For this review, take the finished solid that the model builds, in its own axes (mm). A direction names the side the tool comes from. Coordinates: 2 decimals unless noted, no trailing zeros. Loops run counter-clockwise (first coordinate to the right, second up) from the corner with the lowest first, then second, coordinate; pieces in that order, holes last. Notation, with made-up numbers: (-11.75, 43.25) -> (7.25, 43.25) arc R21 cw to (7.25, 62.25) -> close; hole circle Ø4 at (51.25, 57). An arc over 180 degrees is marked (long way). Use a Markdown table: item, result.
from build123d import *

# Parameters (mm, degrees)
SKETCH2_R           = 150.026309836
BOSS_EXTRUDE1_DEPTH = 7
SKETCH3_W           = 125
SKETCH3_H           = 115
BOSS_EXTRUDE2_DEPTH = 185
SKETCH4_W           = 315
SKETCH4_H           = 250
BOSS_EXTRUDE3_DEPTH = 11
SKETCH5_R           = 28.662420382
BOSS_EXTRUDE4_DEPTH = 790
SKETCH6_W           = 690
SKETCH6_H           = 450
BOSS_EXTRUDE5_DEPTH = 18
SKETCH7_R           = 29.971446918
BOSS_EXTRUDE6_DEPTH = 50
BOSS_EXTRUDE7_DEPTH = 22
BOSS_EXTRUDE8_DEPTH = 37
FILLET1_R           = 10


with BuildPart() as part:
    # Sketch2 → Boss-Extrude1 (new body)
    with BuildSketch(Plane(origin=(0, 0, 0), x_dir=(1, 0, 0), z_dir=(0, 1, 0))):
        with Locations(Location((0, 0, 0), (0, 0, 270))):
            Circle(SKETCH2_R)
    extrude(amount=-BOSS_EXTRUDE1_DEPTH)

    # Sketch3 → Boss-Extrude2 (add)
    with BuildSketch(Plane.XZ.offset(7)):
        Rectangle(SKETCH3_W, SKETCH3_H)
    extrude(amount=BOSS_EXTRUDE2_DEPTH)

    # Sketch4 → Boss-Extrude3 (add)
    with BuildSketch(Plane.XZ.offset(192)):
        Rectangle(SKETCH4_W, SKETCH4_H)
    extrude(amount=BOSS_EXTRUDE3_DEPTH)

    # Sketch5 → Boss-Extrude4 (add)
    with BuildSketch(Plane.XZ.offset(203)):
        with Locations(Location((0, 0, 0), (0, 0, 90))):
            Circle(SKETCH5_R)
    extrude(amount=BOSS_EXTRUDE4_DEPTH)

    # Sketch6 → Boss-Extrude5 (add)
    with BuildSketch(Plane.XZ.offset(993)):
        Rectangle(SKETCH6_W, SKETCH6_H)
    extrude(amount=BOSS_EXTRUDE5_DEPTH)

    # Sketch7 → Boss-Extrude6 (add)
    with BuildSketch(Plane.XZ.offset(1011)):
        with Locations(Location((-295, 175, 0), (0, 0, 270))):
            Circle(SKETCH7_R)
        with Locations(Location((-295, -175, 0), (0, 0, 270))):
            Circle(SKETCH7_R)
        with Locations(Location((295, 175, 0), (0, 0, 270))):
            Circle(SKETCH7_R)
        with Locations(Location((295, -175, 0), (0, 0, 270))):
            Circle(SKETCH7_R)
    extrude(amount=BOSS_EXTRUDE6_DEPTH)

    # Sketch11 → Boss-Extrude7 (add)
    with BuildSketch(Plane(origin=(0, -423, 0), x_dir=(-1, 0, 0), z_dir=(0, -1, 0))):
        Polygon((28.709807748, 0), (28.709807748, -80), (-171.290192252, -80), (-171.290192252, 80), (28.709807748, 80), align=None)
    extrude(amount=BOSS_EXTRUDE7_DEPTH)

    # Sketch12 → Boss-Extrude8 (add)
    with BuildSketch(Plane.XY.offset(80)):
        with BuildLine():
            Line((-77.568003655, -253), (28.662420382, -423))
            ThreePointArc((28.662420382, -423), (-109.452791637, -391.115212019), (-77.568003655, -253))
        make_face()
    boss_extrude8 = extrude(amount=-BOSS_EXTRUDE8_DEPTH)

    # Mirror1: Boss-Extrude8 across plane
    add(boss_extrude8.mirror(Plane.XY))

    # Fillet1
    fillet1_edges = [part.edges().sort_by_distance(p)[0] for p in [
        (-157.5, -197.5, 125),
        (-157.5, -197.5, -125),
        (157.5, -197.5, -125),
        (157.5, -197.5, 125),
    ]]
    fillet(fillet1_edges, radius=FILLET1_R)


solid = part.part
(1) Take a section at A-A on z = -175. Write out the cut boundary in (x, y), plus the area to 3 significant figures.
Found:
| item | result |
|---|---|
| outline | (-345, -1011) -> (-324.97, -1011) -> (-324.97, -1061) -> (-265.03, -1061) -> (-265.03, -1011) -> (265.03, -1011) -> (265.03, -1061) -> (324.97, -1061) -> (324.97, -1011) -> (345, -1011) -> (345, -993) -> (-345, -993) -> close |
| area | 18,400 mm^2 |
(2) Take a section at B-B on x = 295. Write out the cut boundary in (y, z).
Found:
| item | result |
|---|---|
| outline | (-1061, -204.97) -> (-1011, -204.97) -> (-1011, -225) -> (-993, -225) -> (-993, 225) -> (-1011, 225) -> (-1011, 204.97) -> (-1061, 204.97) -> (-1061, 145.03) -> (-1011, 145.03) -> (-1011, -145.03) -> (-1061, -145.03) -> close |
(3) Mouldability with a two-part tool opening along Z and no side actions: class faces 4 (the face through (-25.196, -336.81, 61.759)), 5 (the face through (92, -423, -1)), 6 (the face through (-1, -98, -57.5)) as pulls with the +Z half, pulls with the -Z half, needs draft (parallel to the pull), parting line crosses it, or undercut.
Found:
| item | result |
|---|---|
| face 4 | needs draft |
| face 5 | undercut |
| face 6 | pulls with the -Z half |
(4) For pin 1 Ø9 at (x, y) = (-59, -198.5) entering from -Z; pin 2 Ø8 at (x, z) = (149.5, 169.5) entering from -Y; pin 3 Ø17.5 at (y, z) = (-438, 15.5) entering from -X, all flat-tipped, find the tip position at first contact; note any pin that passes through.
Found:
| item | result |
|---|---|
| pin 1 | stops at z = -125 |
| pin 2 | stops at y = -1011 |
| pin 3 | stops at x = -28.71 |
(5) Take a section at D-D on x = -109.5. Write out the cut boundary in (y, z), plus the area to 3 significant figures.
Found:
| item | result |
|---|---|
| outline | (-1011, -225) -> (-993, -225) -> (-993, 225) -> (-1011, 225) -> close; (-391.04, -80) -> (-284.96, -80) -> (-284.96, -43) -> (-391.04, -43) -> close; (-391.04, 43) -> (-284.96, 43) -> (-284.96, 80) -> (-391.04, 80) -> close; (-203, -125) -> (-192, -125) -> (-192, 125) -> (-203, 125) -> close; (-7, -102.56) -> (0, -102.56) -> (0, 102.56) -> (-7, 102.56) -> close |
| area | 20,100 mm^2 |
(6) For line 1 along Y through (x, z) = (148, 53); line 2 along Y through (x, z) = (135.5, 112); line 3 along Y through (x, z) = (-51.5, -3), list the stretches that pass through material, from the lowest coordinate up.
Found:
| item | result |
|---|---|
| line 1 | y = -1011 to -993, -445 to -423, -203 to -192 |
| line 2 | y = -1011 to -993, -203 to -192 |
| line 3 | y = -1011 to -993, -203 to 0 |
(7) Take a section at C-C on z = 92. Write out the cut boundary in (x, y).
Found:
| item | result |
|---|---|
| outline | (-345, -1011) -> (345, -1011) -> (345, -993) -> (-345, -993) -> close; (-157.5, -203) -> (157.5, -203) -> (157.5, -192) -> (-157.5, -192) -> close; (-118.51, -7) -> (118.51, -7) -> (118.51, 0) -> (-118.51, 0) -> close |
(8) For faces 1 (the face through (2, -7, 65)), 2 (the face through (171.29, -434, 1)), 3 (the face through (-269.728, -1035.65, 158.888)), list the 3-axis set-ups (+Z, -Z, +X, -X, +Y, -Y) from which the entire face can be reached by the end or side of a thin tool; tool diameter is ignored.
Found:
| item | result |
|---|---|
| face 1 | none |
| face 2 | +Z, -Z, +X, +Y |
| face 3 | -Y |
